The listing builds one solid part. Answer for the finished solid, in the listing's coordinates (mm). Face numbers are marked on the shaded views. A direction names the side the tool comes from. Round coordinates to 2 decimals unless told otherwise and drop trailing zeros. Order: outer loops, then holes, each group sorted by start corner. A loop starts at its lowest first (then second) coordinate and runs counter-clockwise, first axis right, second up. Notation, with made-up numbers: M 77,59 L 84,59 A12 ccw 84,65 Z; hole C 78.25,-18.5 d8. An arc over 180 degrees is marked long. Write item = value, one per line. Start each with the question number.
(1) A cutting plane is placed at A-A, the plane z = 0. Determine the outline of the cut face in (x, y).
(2) Straight lines are drawn through the part: probe 1 along X at (y, z) = (3.1, 0); probe 2 along Y at (x, z) = (0, -3.5); probe 3 along X at (y, z) = (19, 3.5). For each, find the intervals that lie inside material, in ascending order. Write a range as from..to.
(3) Which of the six approach directions +Z, -Z, +X, -X, +Y, -Y give full straight-line access (tool end or side, diameter ignored) to the marked faces 1, 2 and 3?
(4) A cutting plane is placed at C-C, the plane z = 6. Determine the outline of the cut face in (x, y).
(5) A cutting plane is placed at B-B, the plane x = -26.5. Determine the outline of the cut face in (y, z), and give its area (3 significant figures).
(6) Each of these flat-tipped pins is pushed along its axis until it touches: pin 1 (4 mm diameter, centred on x = -9.5, z = 1.5, fed in from +Y); pin 2 (3 mm diameter, centred on x = 6.5, z = -1, fed in from +Y); pin 3 (7 mm diameter, centred on x = -25, z = 3, fed in from +Y). Where does it stop, or does it pass through?
(7) A cutting plane is placed at D-D, the plane y = 18. Determine the outline of the cut face in (x, z), and give its area (3 significant figures).
(8) For a pull along Z with two mould halves and no side action, classify the marked faces 4, 5 and 6 as released by +Z, released by -Z, zero draft, split by the parting line, or undercut.
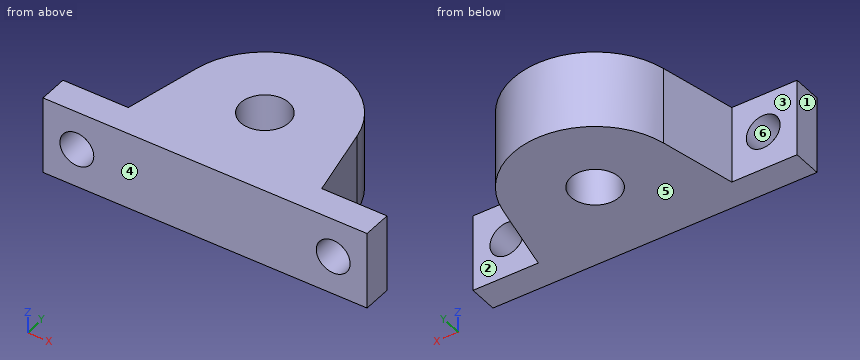
from build123d import *

# Parameters (mm, degrees)
EXTRUDE_1_DEPTH     = 8
SKETCH_2_R          = 3.5
CUT_EXTRUDE_1_DEPTH = 16
SKETCH_3_R          = 5
CUT_EXTRUDE_2_DEPTH = 16


with BuildPart() as part:
    # 草图1 → 凸台-拉伸1 (new body, symmetric)
    with BuildSketch(Plane.XY):
        with BuildLine():
            Line((-33.5, 0), (33.5, 0))
            Line((33.5, 0), (33.5, 6))
            Line((33.5, 6), (20, 6))
            Line((20, 6), (16.613269784, 21.605449639))
            ThreePointArc((16.613269784, 21.605449639), (0, 35), (-16.613269784, 21.605449639))
            Line((-16.613269784, 21.605449639), (-20, 6))
            Line((-20, 6), (-33.5, 6))
            Line((-33.5, 6), (-33.5, 0))
        make_face()
    extrude(amount=EXTRUDE_1_DEPTH, both=True)

    # 草图2 → 切除-拉伸1 (cut)
    with BuildSketch(Plane(origin=(0, 6, 0), x_dir=(1, 0, 0), z_dir=(0, 1, 0))):
        with Locations((-26.5, 0)):
            Circle(SKETCH_2_R)
        with Locations((26.5, 0)):
            Circle(SKETCH_2_R)
    extrude(amount=-CUT_EXTRUDE_1_DEPTH, mode=Mode.SUBTRACT)

    # 草图3 → 切除-拉伸2 (cut)
    with BuildSketch(Plane.XY.offset(8)):
        with Locations((0, 18)):
            Circle(SKETCH_3_R)
    extrude(amount=-CUT_EXTRUDE_2_DEPTH, mode=Mode.SUBTRACT)


solid = part.part
Reported:
q1.outline = M -33.5,0 L -30,0 L -30,6 L -33.5,6 Z; M -23,0 L 23,0 L 23,6 L 20,6 L 16.61,21.61 A17 ccw -16.61,21.61 L -20,6 L -23,6 Z; M 30,0 L 33.5,0 L 33.5,6 L 30,6 Z; hole C 0,18 d10
q2.probe_1 = -33.5..-30, -23..23, 30..33.5
q2.probe_2 = 0..13, 23..35
q2.probe_3 = -17.18..-4.9, 4.9..17.18
q3.face_1 = +Z, -Z, -X, +Y, -Y
q3.face_2 = +Z, -Z, +X, +Y
q3.face_3 = +Z, -Z, -X, +Y
q4.outline = M -33.5,0 L 33.5,0 L 33.5,6 L 20,6 L 16.61,21.61 A17 ccw -16.61,21.61 L -20,6 L -33.5,6 Z; hole C 0,18 d10
q5.outline = M 0,-8 L 6,-8 L 6,-3.5 L 0,-3.5 Z; M 0,3.5 L 6,3.5 L 6,8 L 0,8 Z
q5.area = 54.0 mm²
q6.pin_1 = 33.26
q6.pin_2 = 34.25
q6.pin_3 = 6
q7.outline = M -17.4,-8 L -5,-8 L -5,8 L -17.4,8 Z; M 5,-8 L 17.4,-8 L 17.4,8 L 5,8 Z
q7.area = 397 mm²
q8.face_4 = zero draft
q8.face_5 = released by -Z
q8.face_6 = undercut
